Part model, mm, in its own coordinate system. A direction names the side the tool comes from. Round coordinates to 2 decimals unless told otherwise and drop trailing zeros. Loops run counter-clockwise (first coordinate to the right, second up) from the corner with the lowest first, then second, coordinate; pieces in that order, holes last. Notation, with made-up numbers: (85.25, 50.5) -> (98.25, 50.5) arc R19 ccw to (98.25, 63.5) -> close; hole circle Ø1 at (58.25, 29). An arc over 180 degrees is marked (long way). Answer as CSV lines item,"result".
from build123d import *

# Parameters (mm, degrees)
F0_R     = 8.25
F0_R_2   = 1.6
F1_DEPTH = 8
F2_DEPTH = 3


with BuildPart() as f1:
    # F0 (on Top) → F1 (new body)
    with BuildSketch(Plane.XY):
        with BuildLine():
            Line((-23, -29.708343), (23, -29.708343))
            Line((23, -29.708343), (23, -23.291657))
            ThreePointArc((23, -23.291657), (22.707107, -22.58455), (22, -22.291657))
            Line((22, -22.291657), (8, -22.291657))
            ThreePointArc((8, -22.291657), (7.292893, -21.998763), (7, -21.291657))
            Line((7, -21.291657), (7, -16))
            ThreePointArc((7, -16), (8.464466, -12.464466), (12, -11))
            Line((12, -11), (22, -11))
            ThreePointArc((22, -11), (22.707107, -10.707107), (23, -10))
            Line((23, -10), (23, 6))
            Line((23, 6), (19, 6))
            ThreePointArc((19, 6), (18.292893, 6.292893), (18, 7))
            Line((18, 7), (18, 11))
            Line((18, 11), (-22, 11))
            ThreePointArc((-22, 11), (-22.707107, 10.707107), (-23, 10))
            Line((-23, 10), (-23, -6))
            Line((-23, -6), (-19, -6))
            ThreePointArc((-19, -6), (-18.292893, -6.292893), (-18, -7))
            Line((-18, -7), (-18, -11))
            Line((-18, -11), (-12, -11))
            ThreePointArc((-12, -11), (-8.464466, -12.464466), (-7, -16))
            Line((-7, -16), (-7, -21.291657))
            ThreePointArc((-7, -21.291657), (-7.292893, -21.998763), (-8, -22.291657))
            Line((-8, -22.291657), (-22, -22.291657))
            ThreePointArc((-22, -22.291657), (-22.707107, -22.58455), (-23, -23.291657))
            Line((-23, -23.291657), (-23, -29.708343))
        make_face()
        with Locations((-12.7, 0)):
            Circle(F0_R, mode=Mode.SUBTRACT)
        with Locations((12.7, 0)):
            Circle(F0_R, mode=Mode.SUBTRACT)
        with BuildLine():
            Line((19, 6), (23, 6))
            Line((23, 6), (23, 10))
            ThreePointArc((23, 10), (22.707107, 10.707107), (22, 11))
            Line((22, 11), (18, 11))
            Line((18, 11), (18, 7))
            ThreePointArc((18, 7), (18.292893, 6.292893), (19, 6))
        make_face()
        with Locations((20.5, 8.5)):
            Circle(F0_R_2, mode=Mode.SUBTRACT)
        with BuildLine():
            Line((-22, -11), (-18, -11))
            Line((-18, -11), (-18, -7))
            ThreePointArc((-18, -7), (-18.292893, -6.292893), (-19, -6))
            Line((-19, -6), (-23, -6))
            Line((-23, -6), (-23, -10))
            ThreePointArc((-23, -10), (-22.707107, -10.707107), (-22, -11))
        make_face()
        with Locations((-20.5, -8.5)):
            Circle(F0_R_2, mode=Mode.SUBTRACT)
    extrude(amount=F1_DEPTH)

    # F0 (on Top) → F2 (join)
    with BuildSketch(Plane.XY):
        with BuildLine():
            Line((-22, -11), (-18, -11))
            Line((-18, -11), (-18, -7))
            ThreePointArc((-18, -7), (-18.292893, -6.292893), (-19, -6))
            Line((-19, -6), (-23, -6))
            Line((-23, -6), (-23, -10))
            ThreePointArc((-23, -10), (-22.707107, -10.707107), (-22, -11))
        make_face()
        with Locations((-20.5, -8.5)):
            Circle(F0_R_2, mode=Mode.SUBTRACT)
        with BuildLine():
            Line((19, 6), (23, 6))
            Line((23, 6), (23, 10))
            ThreePointArc((23, 10), (22.707107, 10.707107), (22, 11))
            Line((22, 11), (18, 11))
            Line((18, 11), (18, 7))
            ThreePointArc((18, 7), (18.292893, 6.292893), (19, 6))
        make_face()
        with Locations((20.5, 8.5)):
            Circle(F0_R_2, mode=Mode.SUBTRACT)
    extrude(amount=-F2_DEPTH)


solid = f1.part
Q1. Saw through at A-A, the plane z = -0.75. Write the cut outline in (x, y), then the cut area to 3 significant figures.
Geometry results:
outline,"(-23, -10) arc R1 ccw to (-22, -11) -> (-18, -11) -> (-18, -7) arc R1 ccw to (-19, -6) -> (-23, -6) -> close; (18, 7) arc R1 ccw to (19, 6) -> (23, 6) -> (23, 10) arc R1 ccw to (22, 11) -> (18, 11) -> close; hole circle Ø3.2 at (-20.5, -8.5); hole circle Ø3.2 at (20.5, 8.5)"
area,"33.1 mm2"
Q2. Which spindle directions (+Z, -Z, +X, -X, +Y, -Y) get a long thin tool onto all of the face, cutting with end or side? Do faces 4 (the face through (-18.285, -6.301, -1.479)), 5 (the face through (-21, -6, -1)), 6 (the face through (7.301, -22.006, 3.944)), 7 (the face through (-7.285, -21.991, 3.944)). Say none if no direction does.
Geometry results:
face 4,"-Z, +X, +Y"
face 5,"-Z, +X, -X, +Y"
face 6,"+Z, -Z, +X"
face 7,"+Z, -Z, -X"
Q3. Two-plate mould, pull along Y, no slides. Class faces 1 (the face through (21, 6, -1)), 2 (the face through (-7, -19, 4)), 3 (the face through (23, -27, 4)): pulls with the +Y half, pulls with the -Y half, needs draft (parallel to the pull), parting line crosses it, or undercut.
Geometry results:
face 1,"pulls with the -Y half"
face 2,"undercut"
face 3,"needs draft"
Q4. Saw through at D-D, the plane z = 6.25. Write the cut outline in (x, y), then the cut area to 3 significant figures.
Geometry results:
outline,"(-23, -29.71) -> (23, -29.71) -> (23, -23.29) arc R1 ccw to (22, -22.29) -> (8, -22.29) arc R1 cw to (7, -21.29) -> (7, -16) arc R5 cw to (12, -11) -> (22, -11) arc R1 ccw to (23, -10) -> (23, 10) arc R1 ccw to (22, 11) -> (-22, 11) arc R1 ccw to (-23, 10) -> (-23, -10) arc R1 ccw to (-22, -11) -> (-12, -11) arc R5 cw to (-7, -16) -> (-7, -21.29) arc R1 cw to (-8, -22.29) -> (-22, -22.29) arc R1 ccw to (-23, -23.29) -> close; hole circle Ø3.2 at (-20.5, -8.5); hole circle Ø16.5 at (-12.7, 0); hole circle Ø16.5 at (12.7, 0); hole circle Ø3.2 at (20.5, 8.5)"
area,"1,080 mm2"
Q5. Drill centre lines: line 1 along Y through (x, z) = (-12.7, 5.5); line 2 along Y through (x, z) = (-20.5, -0.7); line 3 along Y through (x, z) = (20.5, -2). Where is each one in solid material? Low to high.
Geometry results:
line 1,"-29.71 to -22.29, -11 to -8.25, 8.25 to 11"
line 2,"-11 to -10.1, -6.9 to -6"
line 3,"6 to 6.9, 10.1 to 11"
Q6. Saw through at C-C, the plane x = -12.7. Write the cut outline in (y, z).
Geometry results:
outline,"(-29.71, 0) -> (-22.29, 0) -> (-22.29, 8) -> (-29.71, 8) -> close; (-11, 0) -> (-8.25, 0) -> (-8.25, 8) -> (-11, 8) -> close; (8.25, 0) -> (11, 0) -> (11, 8) -> (8.25, 8) -> close"
Q7. Saw through at B-B, the plane y = 0. Write the cut outline in (x, z), then the cut area to 3 significant figures.
Geometry results:
outline,"(-23, 0) -> (-20.95, 0) -> (-20.95, 8) -> (-23, 8) -> close; (-4.45, 0) -> (4.45, 0) -> (4.45, 8) -> (-4.45, 8) -> close; (20.95, 0) -> (23, 0) -> (23, 8) -> (20.95, 8) -> close"
area,"104 mm2"
Q8. Drop flat-ended pins along their axis: P1, Ø10, axis at x = -12.7, y = 0, coming from the +Z side; P2, Ø1.5, axis at y = 10, z = -1.5, coming from the -X side; P3, Ø6, axis at y = -19.5, z = 2.5, coming from the -X side; P4, Ø20.5, axis at x = -6, y = -18.5, coming from the -Z side. Give the stop position or say it passes through.
Geometry results:
P1,"through"
P2,"x = 18"
P3,"x = -22.61"
P4,"z = 0"
